```python
from build123d import *

# Parameters (mm, degrees)
PAD014_DEPTH                        = 3
SKETCH055_R                         = 1.65
POCKET019_DEPTH                     = 364.282338
POCKET019_DEPTH_BACK                = 367.282338
BODY001003005003003_PLACEMENT_ANGLE = 60
CLONE002_PLACEMENT_ANGLE            = 124


with BuildPart() as part:
    # Sketch052 → Pad014 (new body)
    with BuildSketch(Plane.XY):
        with BuildLine():
            ThreePointArc((152.959511, 127.101705), (84.480895, 180.040089), (0, 198.875477))
            Line((0, 198.875477), (0, 208.875477))
            ThreePointArc((160.650731, 133.492724), (88.728824, 189.092995), (0, 208.875477))
            ThreePointArc((152.959511, 127.101705), (160.000631, 126.451604), (160.650731, 133.492724))
        make_face()
    pad014 = extrude(amount=PAD014_DEPTH)

    # Sketch055 → Pocket019 (cut, two sides)
    with BuildSketch(Plane.XY) as pocket019_sk:
        with Locations((143.11, 145.205847)):
            Circle(SKETCH055_R)
        with BuildLine():
            Line((0, 202.225477), (0, 205.525477))
            ThreePointArc((0, 202.225477), (1.65, 203.875477), (0, 205.525477))
        make_face()
    pocket019 = extrude(amount=-POCKET019_DEPTH, mode=Mode.SUBTRACT) + extrude(pocket019_sk.sketch, amount=POCKET019_DEPTH_BACK, mode=Mode.SUBTRACT)

    # Mirrored019: Pad014, Pocket019 across Sketch052 V_Axis
    add(pad014.mirror(Plane(origin=(0, 0, 0), x_dir=(0, 0, 1), z_dir=(1, 0, 0))))
    add(pocket019.mirror(Plane(origin=(0, 0, 0), x_dir=(0, 0, 1), z_dir=(1, 0, 0))), mode=Mode.SUBTRACT)


with BuildPart() as part_1:
    # Body001003005003003 placement: moved
    add(part.part.rotate(Axis((0, 0, 0), (0, 0, 1)), BODY001003005003003_PLACEMENT_ANGLE))


with BuildPart() as part_2:
    # Clone002 placement: moved
    add(part_1.part.moved(Location((1305, 724, 0))).rotate(Axis((1305, 724, 0), (0, 0, 1)), CLONE002_PLACEMENT_ANGLE))


solid = part_2.part
```
Design review of the part built by this model. Coordinates are the model's own, in mm. Give positions to 0.01 mm unless a question says otherwise; leave off trailing zeros. Order: outer loops, then holes, each group sorted by start corner. A loop starts at its lowest first (then second) coordinate and runs counter-clockwise, first axis right, second up. Notation, with made-up numbers: (-40, 19.5) - (-31, 19.5) arc R25 cw to (-31, 41.5) - close; hole circle Ø7 at (40.25, -26.5). An arc over 180 degrees is marked (long way). Use a Markdown table: item, result. Add a question column.
(1) Add section B-B on z = 2.35. Give the boundary of the cut face in (x, y).
(2) Add section A-A on y = 562.5. Give the boundary of the cut face in (x, z).
(3) Mouldability with a two-part tool opening along X and no side actions: class faces 1 (the face through (1473.34, 609.08, 1.48)), 2 (the face through (1320, 523, 3)), 3 (the face through (1154.29, 586.77, 1.48)) as +X half, -X half, draft (parallel to the pull), parting line (faces both ways), or undercut.
(4) Add section C-C on y = 575.5. Give the boundary of the cut face in (x, z).
(5) Clearance check with flat-ended pins moving along their axes: P1, Ø1, axis at y = 543, z = 1, coming from the +X side; P2, Ø1, axis at y = 562.5, z = 2.5, coming from the +X side. State where each tip first meets the part, or that it passes through.
(6) Wall thickness on probe 1 along X at (y, z) = (568.5, 0.3); probe 2 along X at (y, z) = (545, 2.15); probe 3 along X at (y, z) = (558.5, 0.65): over which ranges is each line inside the solid? List them lowest first. Write a range as [from, to].
(7) Add section D-D on x = 1346. Give the boundary of the cut face in (y, z), then the cut area to 3 significant figures.
Report:
| question | item | result |
|---|---|---|
| 1 | outline | (1154.05, 579.63) arc R208.88 ccw to (1319.57, 515.63) arc R208.88 ccw to (1474.57, 602.04) arc R5 ccw to (1466.45, 607.88) arc R198.88 cw to (1318.87, 525.61) arc R198.88 cw to (1161.28, 586.54) arc R5 ccw to start; hole circle Ø3.3 at (1172.37, 569.17); hole circle Ø3.3 at (1319.22, 520.62); hole circle Ø3.3 at (1457.89, 589.13) |
| 2 | outline | (1172.54, 0) - (1188.94, 0) - (1188.94, 3) - (1172.54, 3) - close; (1421.06, 0) - (1437.46, 0) - (1437.46, 3) - (1421.06, 3) - close |
| 3 | face 1 | parting line |
| 3 | face 2 | draft |
| 3 | face 3 | undercut |
| 4 | outline | (1158.11, 0) - (1172.72, 0) - (1172.72, 3) - (1158.11, 3) - close; (1437.28, 0) - (1451.89, 0) - (1451.89, 3) - (1437.28, 3) - close |
| 5 | P1 | stops at x = 1410.11 |
| 5 | P2 | stops at x = 1438.07 |
| 6 | probe 1 | x = [1165.54, 1170.86], [1173.88, 1181.02], [1428.98, 1444.46] |
| 6 | probe 2 | x = [1197.35, 1218.34], [1391.66, 1412.65] |
| 6 | probe 3 | x = [1177.57, 1194.72], [1415.28, 1432.43] |
| 7 | outline | (519.19, 0) - (529.4, 0) - (529.4, 3) - (519.19, 3) - close |
| 7 | area | 30.6 mm² |
